from build123d import *

# Parameters (mm, degrees)
SKETCH1_W           = 96
SKETCH1_H           = 49
BOSS_EXTRUDE1_DEPTH = 15.494
SKETCH2_W           = 127
SKETCH2_H           = 64.5
BOSS_EXTRUDE2_DEPTH = 1.27
SHELL1_START        = -46.73
SHELL1_OUTLINE_W    = 47.73
SHELL1_OUTLINE_H    = 14.224
SHELL1_DEPTH        = 93.46


# Read off the part's stored shape, not the designer's step: Shell1
with BuildPart() as part:
    # Sketch1 → Boss-Extrude1 (new body)
    with BuildSketch(Plane.XY):
        Rectangle(SKETCH1_W, SKETCH1_H)
    extrude(amount=BOSS_EXTRUDE1_DEPTH)

    # Sketch2 → Boss-Extrude2 (add)
    with BuildSketch(Plane.XY.offset(15.494)):
        with Locations((0, 7.75)):
            Rectangle(SKETCH2_W, SKETCH2_H)
    extrude(amount=-BOSS_EXTRUDE2_DEPTH)

    # Shell1 outline → Shell1 (cut)
    with BuildSketch(Plane.YZ.offset(SHELL1_START)):
        with Locations((-0.635, 8.382)):
            Rectangle(SHELL1_OUTLINE_W, SHELL1_OUTLINE_H)
    extrude(amount=SHELL1_DEPTH, mode=Mode.SUBTRACT)


solid = part.part
Verification items for the finished model (mm, model axes). A direction names the side the tool comes from. Coordinates: 2 decimals unless noted, no trailing zeros. Write each loop counter-clockwise with the first axis right and the second up, starting at its lowest first coordinate (ties: lowest second). Pieces come first, ordered by that corner, then holes. Notation, with made-up numbers: M 15,50 L 39,50 A29 cw 39,81 Z; hole C 49.25,50.25 d6. An arc over 180 degrees is marked long. Use a Markdown table: item, result.
Q1. Sectioned sample at A-A, the plane y = -16.5. Record the boundary of the cut face in (x, z), plus the area to 3 significant figures.
Reply:
| item | result |
|---|---|
| outline | M -63.5,14.22 L -48,14.22 L -48,0 L 48,0 L 48,14.22 L 63.5,14.22 L 63.5,15.49 L 46.73,15.49 L 46.73,1.27 L -46.73,1.27 L -46.73,15.49 L -63.5,15.49 Z |
| area | 197 mm² |
Q2. Go/stop test with flat-tipped pins: P1, Ø4.5, axis at y = -7, z = 5, coming from the -X side; P2, Ø1, axis at x = 35, z = 3, coming from the +Y side; P3, Ø4.5, axis at y = -7, z = 9, coming from the +X side. Record where each tip stops, or that it passes through.
Reply:
| item | result |
|---|---|
| P1 | stops at x = -48 |
| P2 | stops at y = 24.5 |
| P3 | stops at x = 48 |
Q3. Sectioned sample at C-C, the plane z = 12. Record the boundary of the cut face in (x, y).
Reply:
| item | result |
|---|---|
| outline | M -48,-24.5 L -46.73,-24.5 L -46.73,23.23 L 46.73,23.23 L 46.73,-24.5 L 48,-24.5 L 48,24.5 L -48,24.5 Z |
Q4. Sectioned sample at D-D, the plane y = 34.5. Record the boundary of the cut face in (x, z).
Reply:
| item | result |
|---|---|
| outline | M -63.5,14.22 L 63.5,14.22 L 63.5,15.49 L -63.5,15.49 Z |
Q5. Sectioned sample at B-B, the plane x = -33. Record the boundary of the cut face in (y, z).
Reply:
| item | result |
|---|---|
| outline | M -24.5,0 L 24.5,0 L 24.5,14.22 L 40,14.22 L 40,15.49 L 23.23,15.49 L 23.23,1.27 L -24.5,1.27 Z |
Q6. Draft check along X on faces 1 (the face through (-1, -1, 1.27)), 2 (the face through (0, -24.5, 1)), 3 (the face through (48, 0, 7)), 4 (the face through (-48, 0, 7)). Enter one of: +X half, -X half, draft (parallel to the pull), parting line (faces both ways), or undercut.
Reply:
| item | result |
|---|---|
| face 1 | undercut |
| face 2 | draft |
| face 3 | +X half |
| face 4 | -X half |
Q7. Thickness scan on line 1 (X direction, y = -1.5, z = 5.75); line 2 (Y direction, x = 33, z = 1.5); line 3 (Z direction, x = -12, y = 2.5). Record the ranges inside material, lowest first.
Reply:
| item | result |
|---|---|
| line 1 | x = -48 to -46.73, 46.73 to 48 |
| line 2 | y = 23.23 to 24.5 |
| line 3 | z = 0 to 1.27 |
Q8. Set-up check for faces 5 (the face through (-1, 0, 0)), 6 (the face through (-1, 24.5, 7)), 7 (the face through (-46.73, -1, 8)): record each of +Z, -Z, +X, -X, +Y, -Y from which the full face is reachable in a straight line by a thin tool's end or side.
Reply:
| item | result |
|---|---|
| face 5 | -Z, +X, -X, +Y, -Y |
| face 6 | -Z, +X, -X, +Y |
| face 7 | +Z, -Y |
